Could you check a few things on this drawing? It's one solid part, dimensions in mm from its lowest x, y, z. A direction names the side the tool comes from. Round coordinates to 2 decimals unless told otherwise and drop trailing zeros. Loops run counter-clockwise (first coordinate to the right, second up) from the corner with the lowest first, then second, coordinate; pieces in that order, holes last. Notation, with made-up numbers: M -8.5,1 L -3.5,1 A27 cw -3.5,28 Z; hole C 64.25,76.25 d11. An arc over 180 degrees is marked long. Use a Markdown table: item, result. Add a question column.
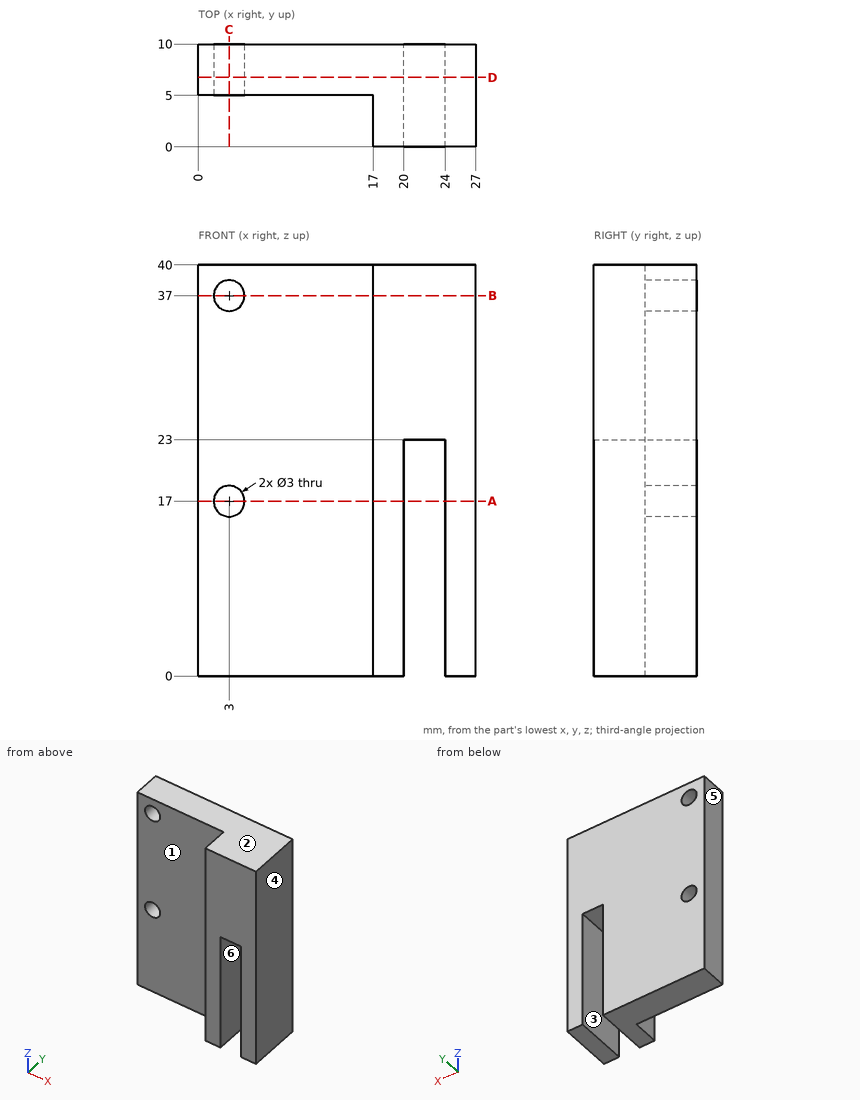
(1) Suppose I cut it at C-C on x = 3. List the corners of the cut face in (y, z) for me, and give its area (3 significant figures).
(2) Suppose I cut it at B-B on z = 37. List the corners of the cut face in (x, y) for me, and give its area (3 significant figures).
(3) Thinking about a two-plate mould opening in X: for the marked faces 4, 5 and 6, which applies, released by +X, released by -X, zero draft, split by the parting line, or undercut?
(4) Suppose I cut it at D-D on y = 6.75. List the corners of the cut face in (x, z) for me, and give its area (3 significant figures).
(5) On a 3-axis mill with a long thin cutter (end or side, diameter ignored), from which of +Z, -Z, +X, -X, +Y, -Y can I reach the whole of each face in a straight line? I mean the marked faces 1, 2 and 3. Say none if no direction works.
(6) I'm going to push flat-ended pins straight in: pin 1 (5 mm diameter, centred on y = 4.5, z = 7.5, fed in from -X); pin 2 (5 mm diameter, centred on x = 9, z = 13, fed in from -Y); pin 3 (1 mm diameter, centred on x = 22.5, y = 2, fed in from -Z); pin 4 (1.5 mm diameter, centred on y = 3, z = 23.5, fed in from -X). Where does each tip first touch, or does it pass through?
(7) Suppose I cut it at A-A on z = 17. List the corners of the cut face in (x, y) for me.
(8) If I drill on probe 1 along Z at (x, y) = (3, 7.6); probe 2 along X at (y, z) = (3, 3.5); probe 3 along Y at (x, z) = (16.25, 20.5), over which ranges is the centre line in solid material (lowest first)? Write a range as [from, to].
Results below:
| question | item | result |
|---|---|---|
| 1 | outline | M 5,0 L 10,0 L 10,15.5 L 5,15.5 Z; M 5,18.5 L 10,18.5 L 10,35.5 L 5,35.5 Z; M 5,38.5 L 10,38.5 L 10,40 L 5,40 Z |
| 1 | area | 170 mm² |
| 2 | outline | M 0,5 L 1.5,5 L 1.5,10 L 0,10 Z; M 4.5,5 L 17,5 L 17,0 L 27,0 L 27,10 L 4.5,10 Z |
| 2 | area | 170 mm² |
| 3 | face 4 | released by +X |
| 3 | face 5 | released by -X |
| 3 | face 6 | undercut |
| 4 | outline | M 0,0 L 20,0 L 20,23 L 24,23 L 24,0 L 27,0 L 27,40 L 0,40 Z; hole C 3,17 d3; hole C 3,37 d3 |
| 4 | area | 974 mm² |
| 5 | face 1 | +Z, -Z, -X, -Y |
| 5 | face 2 | +Z, +X, -X, +Y, -Y |
| 5 | face 3 | -Z, +Y, -Y |
| 6 | pin 1 | stops at x = 0 |
| 6 | pin 2 | stops at y = 5 |
| 6 | pin 3 | stops at z = 23 |
| 6 | pin 4 | stops at x = 17 |
| 7 | outline | M 0,5 L 1.5,5 L 1.5,10 L 0,10 Z; M 4.5,5 L 17,5 L 17,0 L 20,0 L 20,10 L 4.5,10 Z; M 24,0 L 27,0 L 27,10 L 24,10 Z |
| 8 | probe 1 | z = [0, 15.5], [18.5, 35.5], [38.5, 40] |
| 8 | probe 2 | x = [17, 20], [24, 27] |
| 8 | probe 3 | y = [5, 10] |
